The listing builds one solid part. Answer for the finished solid, in the listing's coordinates (mm). Face numbers are marked on the shaded views. A direction names the side the tool comes from. Give positions to 0.01 mm unless a question says otherwise; leave off trailing zeros. Write each loop counter-clockwise with the first axis right and the second up, starting at its lowest first coordinate (ties: lowest second). Pieces come first, ordered by that corner, then holes. Notation, with made-up numbers: (-14, 58) -> (-5, 58) arc R21 ccw to (-5, 93) -> close; hole circle Ø3 at (41, -39.75). An arc over 180 degrees is marked (long way). Put each result on its own line as item: value. Start each with the question number.
1) A cutting plane is placed at D-D (x = 50). Write down the section's boundary in (y, z), then the cut area to 3 significant figures.
2) A cutting plane is placed at C-C (x = 73.5). Write down the section's boundary in (y, z), then the cut area to 3 significant figures.
3) Flat-ended cylindrical pins translate along their axes: pin 1 Ø7 at (x, y) = (-9.39, 137) entering from -Z; pin 2 Ø12 at (y, z) = (107, 49.5) entering from -X; pin 3 Ø3 at (x, z) = (-75.5, 10) entering from +Y. Find the tip coordinate at first contact, or state that the pin passes through.
4) A cutting plane is placed at B-B (y = -38.5). Write down the section's boundary in (x, z).
5) Find the intervals of material crossed by line 1 along Y through (x, z) = (10, 4.5); line 2 along Y through (x, z) = (2, 10); line 3 along Y through (x, z) = (10, 11), in increasing order. Write a range as from..to.
6) A cutting plane is placed at A-A (z = 53.5). Write down the section's boundary in (x, y), then the cut area to 3 significant figures.
7) For a pull along X with two mould halves and no side action, classify the marked faces 1, 2, 3 and 4 as released by +X, released by -X, zero draft, split by the parting line, or undercut.
8) For the marked faces 5, 6 and 7, determine the directions among +Z, -Z, +X, -X, +Y, -Y from which every point of the face is accessible in a straight line to the end or side of a thin tool.
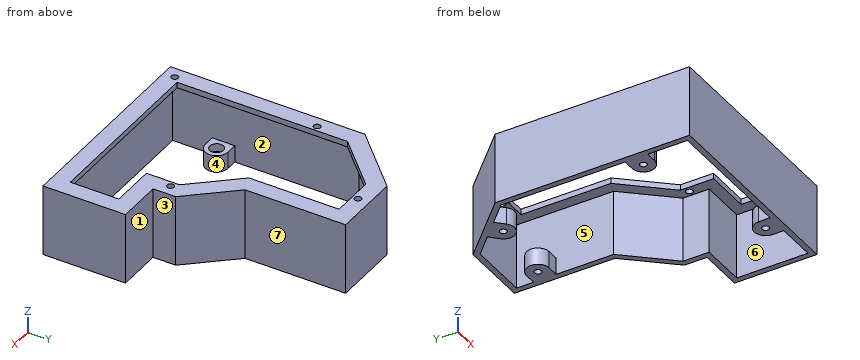
from build123d import *

# Parameters (mm, degrees)
EXTRUDE_1_DEPTH     = 63
SKETCH_2_W          = 185
SKETCH_2_H          = 5
CUT_EXTRUDE_1_DEPTH = 114
SHELL_1_T           = -5
CUT_EXTRUDE_2_DEPTH = 10
EXTRUDE_2_DEPTH     = 15
SKETCH_5_R          = 3
CUT_EXTRUDE_3_DEPTH = 35
SKETCH_6_R          = 6
CUT_EXTRUDE_4_DEPTH = 7
SKETCH_8_R          = 3
CUT_EXTRUDE_5_DEPTH = 10


with BuildPart() as part:
    # 草图1 → 凸台-拉伸1 (new body)
    with BuildSketch(Plane.XY):
        Polygon((100, -2.031815791), (60, -2.031815791), (60, 17.968184209), (25, 57.968184209), (25, 147), (-35, 147), (-85, 97), (-85, -80), (100, -80), align=None)
    extrude(amount=EXTRUDE_1_DEPTH)

    # 草图2 → 切除-拉伸1 (cut)
    with BuildSketch(Plane.XY.offset(63)):
        with Locations((7.5, -77.5)):
            Rectangle(SKETCH_2_W, SKETCH_2_H)
    extrude(amount=-CUT_EXTRUDE_1_DEPTH, mode=Mode.SUBTRACT)

    # 抽壳1
    shell_1_openings = [part.faces().sort_by_distance(p)[0] for p in [
        (18.333333333, 34.763637426, 0),
    ]]
    offset(amount=SHELL_1_T, openings=shell_1_openings, kind=Kind.INTERSECTION)

    # 草图3 → 切除-拉伸2 (cut)
    with BuildSketch(Plane(origin=(0, 0, 58), x_dir=(-1, 0, 0), z_dir=(0, 0, -1))):
        Polygon((-85, -60), (70, -60), (70, 90.786796564), (28.786796564, 132), (-10, 132), (-10, 52.332157467), (-45, 12.332157467), (-45, -17.031815791), (-85, -17.031815791), align=None)
    extrude(amount=-CUT_EXTRUDE_2_DEPTH, mode=Mode.SUBTRACT)

    # 草图4 → 凸台-拉伸2 (add)
    with BuildSketch(Plane(origin=(0, 0, 0), x_dir=(-1, 0, 0), z_dir=(0, 0, -1))):
        with BuildLine():
            Line((63.535533906, 111.393398282), (56.464466094, 104.32233047))
            ThreePointArc((56.464466094, 104.32233047), (42.32233047, 104.32233047), (42.32233047, 118.464466094))
            Line((42.32233047, 118.464466094), (49.393398282, 125.535533906))
            Line((49.393398282, 125.535533906), (63.535533906, 111.393398282))
        make_face()
        with BuildLine():
            Line((70, -15), (80, -15))
            Line((80, -15), (80, -35))
            Line((80, -35), (70, -35))
            ThreePointArc((70, -35), (60, -25), (70, -15))
        make_face()
        with BuildLine():
            Line((-40, -60), (-40, -70))
            Line((-40, -70), (-60, -70))
            Line((-60, -70), (-60, -60))
            ThreePointArc((-60, -60), (-50, -50), (-40, -60))
        make_face()
        with BuildLine():
            Line((-10, 127), (-20, 127))
            Line((-20, 127), (-20, 107))
            Line((-20, 107), (-10, 107))
            ThreePointArc((-10, 107), (0, 117), (-10, 127))
        make_face()
    extrude(amount=-EXTRUDE_2_DEPTH)

    # 草图5 → 切除-拉伸3 (cut)
    with BuildSketch(Plane(origin=(0, 0, 0), x_dir=(-1, 0, 0), z_dir=(0, 0, -1))):
        with Locations((49.393398282, 111.393398282)):
            Circle(SKETCH_5_R)
        with Locations((-10, 117)):
            Circle(SKETCH_5_R)
        with Locations((70, -25)):
            Circle(SKETCH_5_R)
        with Locations((-50, -60)):
            Circle(SKETCH_5_R)
    extrude(amount=-CUT_EXTRUDE_3_DEPTH, mode=Mode.SUBTRACT)

    # 草图6 → 切除-拉伸4 (cut)
    with BuildSketch(Plane.XY.offset(15)):
        with Locations((10, 117)):
            Circle(SKETCH_6_R)
        with Locations((-49.393398282, 111.393398282)):
            Circle(SKETCH_6_R)
        with Locations((50, -60)):
            Circle(SKETCH_6_R)
        with Locations((-70, -25)):
            Circle(SKETCH_6_R)
    extrude(amount=-CUT_EXTRUDE_4_DEPTH, mode=Mode.SUBTRACT)

    # 草图8 → 切除-拉伸5 (cut)
    with BuildSketch(Plane.XY.offset(63)):
        with Locations((-9.393398282, 137)):
            Circle(SKETCH_8_R)
        with Locations((-75, -65)):
            Circle(SKETCH_8_R)
        with Locations((-75, 60.786796564)):
            Circle(SKETCH_8_R)
        with Locations((50, 7.332157467)):
            Circle(SKETCH_8_R)
    extrude(amount=-CUT_EXTRUDE_5_DEPTH, mode=Mode.SUBTRACT)


solid = part.part
Reply:
1. outline: (-75, 0) -> (-63, 0) -> (-63, 8) -> (-66, 8) -> (-66, 15) -> (-70, 15) -> (-70, 58) -> (-60, 58) -> (-60, 63) -> (-75, 63) -> close; (-57, 0) -> (-50, 0) -> (-50, 15) -> (-54, 15) -> (-54, 8) -> (-57, 8) -> close; (-17.03, 58) -> (4.33, 58) -> (4.33, 63) -> (-17.03, 63) -> close; (10.33, 58) -> (21.8, 58) -> (21.8, 0) -> (29.4, 0) -> (29.4, 63) -> (10.33, 63) -> close
1. area: 1,180 mm2
2. outline: (-75, 0) -> (-70, 0) -> (-70, 58) -> (-60, 58) -> (-60, 63) -> (-75, 63) -> close; (-17.03, 58) -> (-7.03, 58) -> (-7.03, 0) -> (-2.03, 0) -> (-2.03, 63) -> (-17.03, 63) -> close
2. area: 730 mm2
3. pin 1: stops at z = 58
3. pin 2: stops at x = -81
3. pin 3: stops at y = 108
4. outline: (-85, 0) -> (-80, 0) -> (-80, 58) -> (-70, 58) -> (-70, 63) -> (-85, 63) -> close; (85, 58) -> (95, 58) -> (95, 0) -> (100, 0) -> (100, 63) -> (85, 63) -> close
5. line 1: y = -75..-70, 107..114, 120..127, 142..147
5. line 2: y = -75..-70, 111..123, 142..147
5. line 3: y = -75..-70, 107..111, 123..127, 142..147
6. outline: (-85, -75) -> (100, -75) -> (100, -2.03) -> (60, -2.03) -> (60, 17.97) -> (25, 57.97) -> (25, 147) -> (-35, 147) -> (-85, 97) -> close; hole (-80, -70) -> (95, -70) -> (95, -7.03) -> (55, -7.03) -> (55, 16.09) -> (20, 56.09) -> (20, 142) -> (-32.93, 142) -> (-80, 94.93) -> close
6. area: 3,720 mm2
7. face 1: zero draft
7. face 2: undercut
7. face 3: released by +X
7. face 4: undercut
8. face 5: none
8. face 6: -Z
8. face 7: +Z, -Z, +X, +Y
